Autodesk Inventor part; units mm, degrees
ref_plane "YZ Plane" through (0, 0, 0) normal (1, 0, 0) x (0, 1, 0)
ref_plane "XZ Plane" through (0, 0, 0) normal (0, 1, 0) x (-1, 0, 0)
ref_plane "XY Plane" through (0, 0, 0) normal (0, 0, 1) x (1, 0, 0)
sketch "Sketch1" plane through (0, 0, 0) normal (0, 0, 1) x (1, 0, 0)
  line L0 (-292.1, 381) -> (292.1, 381)
  line L1 (292.1, 381) -> (292.1, -381)
  line L2 (292.1, -381) -> (-292.1, -381)
  line L3 (-292.1, -381) -> (-292.1, 381)
  point P0 (0, 0)
  point P1 (0, 381)
  point P2 (292.1, 0)
  dimension "d0" = 584.2
  dimension "d1" = 762
extrude "Extrusion1" add sketch "Sketch1" along normal blind 3
sketch "Sketch2" plane through (0, 0, 3) normal (0, 0, 1) x (1, 0, 0)
  line L0 (292.1, 381) -> (292.1, -381)
  line L1 (292.1, -381) -> (-292.1, -381)
  line L2 (-63.5, 292.1) -> (241.3, 292.1)
  line L3 (241.3, 292.1) -> (241.3, -279.4)
  line L4 (241.3, -279.4) -> (-63.5, -279.4)
  line L5 (-63.5, -279.4) -> (-63.5, 292.1)
  point P0 (0, 0)
  dimension "d4" = 50.8
  dimension "d5" = 101.6
  dimension "d6" = 571.5
  dimension "d7" = 304.8
extrude "Extrusion2" cut sketch "Sketch2" against normal blind 3
properties part number "Left Side"
Here's how the part is built. I have some questions about the finished solid (model axes, mm). Round coordinates to 2 decimals unless told otherwise and drop trailing zeros. Write each loop counter-clockwise with the first axis right and the second up, starting at its lowest first coordinate (ties: lowest second). Pieces come first, ordered by that corner, then holes.
1. Suppose I cut it at A-A (x = 168). List the corners of the cut face in (y, z) for me, and give its area (4 significant figures).
2. I need wall thicknesses on L1, parallel to X at y = 43, z = 1; L2, parallel to Y at x = 181.5, z = 2.1. Which ranges of each line are inside material? Lowest first, please.
3. Suppose I cut it at C-C (z = 1.75). List the corners of the cut face in (x, y) for me.
4. Will this pin go through, and if not, where does the flat tip stop? pin 1 Ø1 at (x, y) = (-208.5, -61) entering from -Z.
5. Suppose I cut it at B-B (y = -197.5). List the corners of the cut face in (x, z) for me.
Answer sheet:
1. outline: (-381, 0) - (-279.4, 0) - (-279.4, 3) - (-381, 3) - close; (292.1, 0) - (381, 0) - (381, 3) - (292.1, 3) - close
1. area: 571.5 mm2
2. L1: x = -292.1 to -63.5, 241.3 to 292.1
2. L2: y = -381 to -279.4, 292.1 to 381
3. outline: (-292.1, -381) - (292.1, -381) - (292.1, 381) - (-292.1, 381) - close; hole (-63.5, -279.4) - (241.3, -279.4) - (241.3, 292.1) - (-63.5, 292.1) - close
4. pin 1: stops at z = 0
5. outline: (-292.1, 0) - (-63.5, 0) - (-63.5, 3) - (-292.1, 3) - close; (241.3, 0) - (292.1, 0) - (292.1, 3) - (241.3, 3) - close
